from build123d import *

# Parameters (mm, degrees)
CIRPATTERN1_COUNT = 6
CHAMFER2_SIZE     = 1.27
CHAMFER3_SIZE     = 0.762


with BuildPart() as part:
    # Sketch1 → Revolve1 (revolve)
    with BuildSketch(Plane.XY, mode=Mode.PRIVATE) as revolve1_sk:
        Polygon((-46.0375, -2.425), (-25.3873, -2.425), (-25.3873, -5.6), (-10, -5.6), (-10, 5.6), (-46.0375, 5.6), align=None)
    revolve(revolve1_sk.sketch.rotate(Axis((0, -8.7159552, 0), (0, 1, 0)), 180), axis=Axis((0, -8.7159552, 0), (0, 1, 0)))  # turned: the seam where the file's is

    # Sketch2 → 3_8 Clearance Hole1 (revolve, cut)
    with BuildSketch(Plane(origin=(34.925, 5.6, 0), x_dir=(0, 0, 1), z_dir=(1, 0, 0))):
        Polygon((0, 0), (0, 8.025), (5.842, 8.025), (5.15874, 7.238999282), (5.15874, 0.786000718), (5.842, 0), align=None)
    f_3_8_clearance_hole1 = revolve(axis=Axis((34.925, 11.95, 0), (0, -1, 0)), mode=Mode.SUBTRACT)

    # CirPattern1: 3_8 Clearance Hole1 ×6 about axis
    cirpattern1_axis = Axis((0, 0, 0), (0, 1, 0))
    for i in range(1, CIRPATTERN1_COUNT):
        add(f_3_8_clearance_hole1.rotate(cirpattern1_axis, i * 360 / CIRPATTERN1_COUNT), mode=Mode.SUBTRACT)

    # Chamfer2
    chamfer2_edges = [part.edges().sort_by_distance(p)[0] for p in [
        (-10, -5.6, 0),
    ]]
    chamfer(chamfer2_edges, length=CHAMFER2_SIZE)

    # Chamfer3
    chamfer3_edges = [part.edges().sort_by_distance(p)[0] for p in [
        (-25.3873, -5.6, 0),
        (-46.0375, -2.425, 0),
        (-46.0375, 5.6, 0),
        (-10, 5.6, 0),
    ]]
    chamfer(chamfer3_edges, length=CHAMFER3_SIZE)


solid = part.part
Geometry: final body of the model. Coordinates: model frame, mm. Give positions to 0.01 mm unless a question says otherwise; leave off trailing zeros. Order: outer loops, then holes, each group sorted by start corner. A loop starts at its lowest first (then second) coordinate and runs counter-clockwise, first axis right, second up. Notation, with made-up numbers: (-10, 57) -> (32, 57) arc R37 ccw to (32, 93) -> close; hole circle Ø10 at (-11.75, 49). An arc over 180 degrees is marked (long way). Answer as a JSON object with one key per item and string values.
Q1. First-contact query: pin 1 (16.5 mm diameter, centred on x = -34.925, z = 0, fed in from -Y) (3 decimals); pin 2 (1 mm diameter, centred on x = -36.5, y = 4, fed in from +Z); pin 3 (1 mm diameter, centred on y = 1.5, z = 17.5, fed in from -X). Flat tips, straight axial feed; report the tip coordinate or a pass-through.
Entries:
{"pin 1": "stops at y = -2.425", "pin 2": "stops at z = 28.7", "pin 3": "stops at x = -42.78"}
Q2. Draft query along X for faces 1 (the flat face through (19, -2.425, 19)), 2 (the cylindrical face through (-5.503, -3.648, 24.784)), 3 (the cylindrical face through (-33.38, 1.63, -4.92)). Return one class per face: released by +X, released by -X, zero draft, split by the parting line, or undercut.
Entries:
{"face 1": "zero draft", "face 2": "split by the parting line", "face 3": "undercut"}
Q3. Section A-A (x = 0). Output: boundary loops of the cut face in (y, z) (1 decimal).
Entries:
{"outline": "(-5.6, -24.6) -> (-4.8, -25.4) -> (-2.4, -25.4) -> (-2.4, -45.3) -> (-1.7, -46) -> (4.8, -46) -> (5.6, -45.3) -> (5.6, -10.8) -> (4.8, -10) -> (-4.3, -10) -> (-5.6, -11.3) -> close; (-5.6, 11.3) -> (-4.3, 10) -> (4.8, 10) -> (5.6, 10.8) -> (5.6, 45.3) -> (4.8, 46) -> (-1.7, 46) -> (-2.4, 45.3) -> (-2.4, 25.4) -> (-4.8, 25.4) -> (-5.6, 24.6) -> close"}
Q4. Material intervals for probe 1 along Z at (x, y) = (0, 1); probe 2 along X at (y, z) = (-1.75, 32); probe 3 along X at (y, z) = (3.75, 3), sorted ascending.
Entries:
{"probe 1": "z = -46.04 to -10, 10 to 46.04", "probe 2": "x = -32.98 to -22.42, -12.51 to 12.51, 22.42 to 32.98", "probe 3": "x = -45.94 to -39.12, -30.73 to -9.54, 9.54 to 30.73, 39.12 to 45.94"}
Q5. Section B-B (y = 2). Output: boundary loops of the cut face in (x, z) (1 decimal), plus the area to 3 significant figures.
Entries:
{"outline": "circle Ø92.1 at (0, 0); hole circle Ø10.3 at (-34.9, 0); hole circle Ø10.3 at (-17.5, -30.2); hole circle Ø10.3 at (-17.5, 30.2); hole circle Ø20 at (0, 0); hole circle Ø10.3 at (17.5, -30.2); hole circle Ø10.3 at (17.5, 30.2); hole circle Ø10.3 at (34.9, 0)", "area": "5,840 mm^2"}
Q6. Section C-C (z = 0). State how many separate pieces and enclosed holes the cut face has, plus the area to 3 significant figures.
Entries:
{"separate pieces": "4", "enclosed holes": "0", "area": "504 mm^2"}
